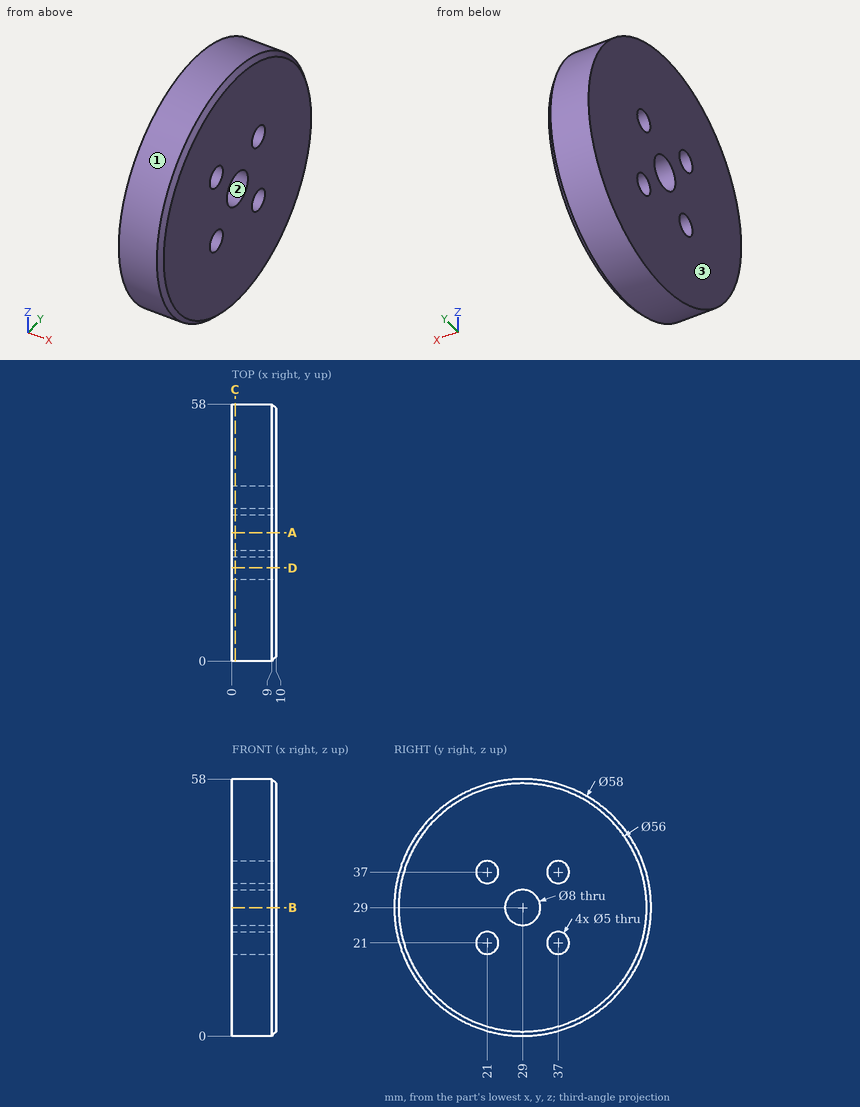
Design review of the part shown in the three views and the two pictorial views. Dimensions are in mm from the part's minimum x, y and z. Round coordinates to 2 decimals unless told otherwise and drop trailing zeros. Loops run counter-clockwise (first coordinate to the right, second up) from the corner with the lowest first, then second, coordinate; pieces in that order, holes last. Notation, with made-up numbers: (-7.5, 45) - (22.5, 45) arc R16 cw to (22.5, 72) - close; hole circle Ø4 at (80, -19). An arc over 180 degrees is marked (long way). One line per item, written item: value. Start each with the question number.
Item 1: Take a section at C-C (x = 0.75). Give the boundary of the cut face in (y, z).
Item 2: Clearance check with flat-ended pins moving along their axes: pin 1 Ø2 at (y, z) = (42, 23.5) entering from -X; pin 2 Ø1 at (x, z) = (8, 46) entering from +Y; pin 3 Ø6 at (x, y) = (6, 6) entering from +Z; pin 4 Ø2 at (x, y) = (7.5, 35) entering from +Z. State where each tip first meets the part, or that it passes through.
Item 3: Take a section at D-D (y = 21). State how many separate pieces and enclosed holes the cut face has, plus the area to 3 significant figures.
Item 4: For L1, parallel to Z at x = 5, y = 37; L2, parallel to Z at x = 6.25, y = 35, list the stretches that pass through material, from the lowest coordinate up.
Item 5: Take a section at A-A (y = 29). Give the boundary of the cut face in (x, z), plus the area to 3 significant figures.
Item 6: The part is to be moulded in two halves that separate along Z. For the marked faces 1, 2 and 3, say which applies: +Z half, -Z half, draft (parallel to the pull), parting line (faces both ways), or undercut.
Answer below:
1. outline: circle Ø58 at (29, 29); hole circle Ø5 at (21, 21); hole circle Ø5 at (21, 37); hole circle Ø8 at (29, 29); hole circle Ø5 at (37, 21); hole circle Ø5 at (37, 37)
2. pin 1: stops at x = 0
2. pin 2: stops at y = 52.85
2. pin 3: stops at z = 50
2. pin 4: stops at z = 57.57
3. separate pieces: 3
3. enclosed holes: 0
3. area: 456 mm2
4. L1: z = 1.13 to 18.5, 23.5 to 34.5, 39.5 to 56.87
4. L2: z = 0.63 to 19.5, 22.5 to 35.5, 38.5 to 57.37
5. outline: (0, 0) - (9, 0) - (10, 1) - (10, 25) - (0, 25) - close; (0, 33) - (10, 33) - (10, 57) - (9, 58) - (0, 58) - close
5. area: 499 mm2
6. face 1: parting line
6. face 2: undercut
6. face 3: draft
